Check sheet for the modelled part. Datum: model origin and axes. Units: mm. A direction names the side the tool comes from. Round coordinates to 2 decimals unless told otherwise and drop trailing zeros. Write each loop counter-clockwise with the first axis right and the second up, starting at its lowest first coordinate (ties: lowest second). Pieces come first, ordered by that corner, then holes. Notation, with made-up numbers: M 47,-28.75 L 81,-28.75 A19 ccw 81,-6.75 Z; hole C -16.5,8.5 d4. An arc over 180 degrees is marked long. Answer in a Markdown table with one row per item.
Autodesk Inventor part; units mm, degrees
ref_plane "YZ Plane" through (0, 0, 0) normal (1, 0, 0) x (0, 1, 0)
ref_plane "XZ Plane" through (0, 0, 0) normal (0, 1, 0) x (-1, 0, 0)
ref_plane "XY Plane" through (0, 0, 0) normal (0, 0, 1) x (1, 0, 0)
sketch "Sketch1" plane through (0, 0, 0) normal (0, 1, 0) x (-1, 0, 0)
  line L0 (0, 0) -> (0, 135)
  line L1 (0, 135) -> (0, -135)
  line L2 (0, -135) -> (50, -135)
  line L3 (50, -135) -> (-50, -135)
  line L4 (-50, -135) -> (-50, 135)
  line L5 (-50, 135) -> (50, 135)
  line L6 (50, 135) -> (50, -135)
  line L7 (50, 135) -> (50, 127.5)
  line L8 (50, 127.5) -> (40, 127.5)
  circle A0 centre (40, 127.5) radius 3
  line L9 (40, 127.5) -> (-40, 127.5)
  circle A1 centre (-40, 127.5) radius 3
  line L10 (50, 0) -> (-50, 0)
  circle A2 centre (40, -127.5) radius 3
  circle A3 centre (-40, -127.5) radius 3
  dimension "d0" = 135
  dimension "d1" = 270
  dimension "d2" = 50
  dimension "d3" = 100
  dimension "d4" = 7.5
  dimension "d5" = 10
  dimension "d6" = 6
  dimension "d7" = 80
  dimension "d8" = 6
extrude "Extrusion1" add sketch "Sketch1" along normal blind 5 contours L10 L4 L5 L0 | L10 L6 L2 L1 | L0 L9 A0 L8 L6 L10 | L1 L3 L4 L10 | L0 L5 L6 L8 A0 L9
sketch "Sketch2" plane through (0, 5, 0) normal (0, 1, 0) x (1, 0, 0)
  line L0 (0, 0) -> (50, 0)
  line L1 (50, -135) -> (50, 135)
  line L2 (50, 0) -> (50, 100)
  line L3 (50, 100) -> (0, 100)
  line L4 (0, 100) -> (0, 0)
  dimension "d11" = 100
extrude "Extrusion2" add sketch "Sketch2" along normal blind 15
fillet "Fillet1" radius 5 1 edges at (0, 12.5, -100)
fillet "Fillet2" radius 5 1 edges at (0, 12.5, 0)
sketch "Sketch3" plane through (50, 5, -100) normal (0, 0, -1) x (-1, 0, 0)
  line L0 (0, 0) -> (0, 15)
  line L1 (0, 0) -> (0, 7.5)
  line L2 (0, 7.5) -> (20, 7.5)
  circle A0 centre (20, 7.5) radius 2.5
  point P0 (50, -5)
  dimension "d16" = 7.5
  dimension "d17" = 20
  dimension "d18" = 5
hole "Hole1" at (30, 12.5, -100) direction (0, 0, 1) diameter 6 depth 20 tip angle 118
sketch "Sketch4" plane through (0, 0, 0) normal (0, -1, 0) x (1, 0, 0)
  line L0 (50, -135) -> (-50, -135)
  line L1 (50, -135) -> (33, -135)
  line L2 (33, -135) -> (33, -100)
  line L3 (5, -100) -> (50, -100)
  line L4 (33, -100) -> (40, -100)
  line L5 (40, -100) -> (23, -100)
  line L6 (23, -100) -> (23, -50)
  line L7 (23, -50) -> (40, -50)
  line L8 (40, -50) -> (40, -100)
  line L9 (40, -100) -> (40, -95)
  line L10 (40, -95) -> (23, -95)
  line L11 (23, -95) -> (23, -100)
  point P0 (0, 0)
  dimension "d26" = 17
  dimension "d27" = 35
  dimension "d28" = 7
  dimension "d29" = 17
  dimension "d30" = 50
  dimension "d31" = 5
extrude "Extrusion3" cut sketch "Sketch4" against normal blind 16 contours L6 L7 L8 L10
properties part number "side_front"
1. Scan lines: L1, parallel to Z at x = -40, y = 3.1; L2, parallel to X at y = 11.5, z = -30.5; L3, parallel to X at y = 12.5, z = -97.7. Record each from-to range of solid material in increasing order.
Found:
| item | result |
|---|---|
| L1 | z = -135 to -130.5, -124.5 to 124.5, 130.5 to 135 |
| L2 | x = 0 to 50 |
| L3 | x = 0.79 to 27, 33 to 50 |
2. Access from +Z, -Z, +X, -X, +Y, -Y to the whole of each face (thin tool, end or side, straight path). Record for faces 4 (the face through (40, 8, -72)), 5 (the face through (27, 12, 0)), 6 (the face through (2, 13, -99)), 7 (the face through (28, 9, -100)), 8 (the face through (1, 13, -2)).
Found:
| item | result |
|---|---|
| face 4 | -Y |
| face 5 | +Z, +X, -X, +Y |
| face 6 | -Z, -X, +Y |
| face 7 | -Z, +X, -X, +Y |
| face 8 | +Z, -X, +Y |
3. Section check B-B, the plane z = 127.5. Record the cut outline in (x, y).
Found:
| item | result |
|---|---|
| outline | M -50,0 L -43,0 L -43,5 L -50,5 Z; M -37,0 L 37,0 L 37,5 L -37,5 Z; M 43,0 L 50,0 L 50,5 L 43,5 Z |
4. Section check C-C, the plane y = 2.5. Record the cut outline in (x, z), and give its area (3 significant figures).
Found:
| item | result |
|---|---|
| outline | M -50,-135 L 50,-135 L 50,135 L -50,135 Z; hole C -40,-127.5 d6; hole C -40,127.5 d6; hole M 23,-95 L 40,-95 L 40,-50 L 23,-50 Z; hole C 40,-127.5 d6; hole C 40,127.5 d6 |
| area | 26,100 mm2 |
5. Go/stop test with flat-tipped pins: pin 1 (13.5 mm diameter, centred on x = 30.5, z = -68, fed in from -Y); pin 2 (4.5 mm diameter, centred on y = 14, z = -42, fed in from -X); pin 3 (5.5 mm diameter, centred on x = 40, z = 127.5, fed in from +Y); pin 4 (6 mm diameter, centred on x = 35.5, z = 104.5, fed in from +Y). Record where each tip stops, or that it passes through.
Found:
| item | result |
|---|---|
| pin 1 | stops at y = 16 |
| pin 2 | stops at x = 0 |
| pin 3 | passes through |
| pin 4 | stops at y = 5 |
6. Section check D-D, the plane z = -62.5. Record the cut outline in (x, y).
Found:
| item | result |
|---|---|
| outline | M -50,0 L 23,0 L 23,16 L 40,16 L 40,0 L 50,0 L 50,20 L 0,20 L 0,5 L -50,5 Z |
7. Section check A-A, the plane x = -40. Record the cut outline in (y, z).
Found:
| item | result |
|---|---|
| outline | M 0,-135 L 5,-135 L 5,-130.5 L 0,-130.5 Z; M 0,-124.5 L 5,-124.5 L 5,124.5 L 0,124.5 Z; M 0,130.5 L 5,130.5 L 5,135 L 0,135 Z |
8. Draft check along Z on faces 1 (the face through (1, 2, 135)), 2 (the face through (-1, 2, -135)), 3 (the face through (-37.79, 2.46, 125.47)). Enter one of: +Z half, -Z half, draft (parallel to the pull), parting line (faces both ways), or undercut.
Found:
| item | result |
|---|---|
| face 1 | +Z half |
| face 2 | -Z half |
| face 3 | undercut |
